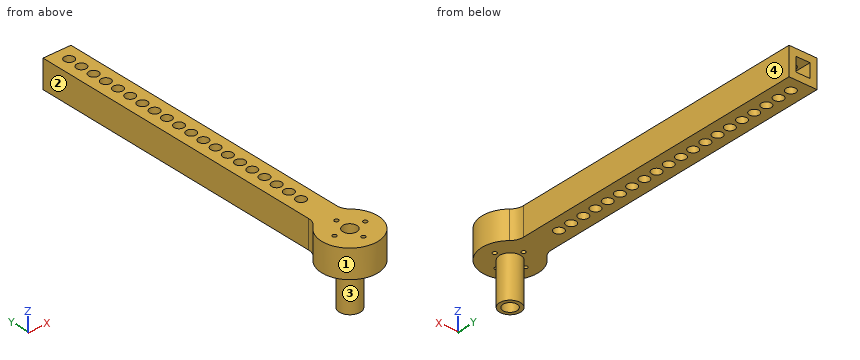
```python
from build123d import *

# Parameters (mm, degrees)
SKETCH1_W           = 12.7
SKETCH1_H           = 12.7
SKETCH1_W_2         = 6.35
SKETCH1_H_2         = 6.35
BOSS_EXTRUDE1_DEPTH = 152.4
SKETCH2_R           = 2.226999991
CUT_EXTRUDE1_DEPTH  = 13.7
SKETCH3_R           = 12.7
BOSS_EXTRUDE2_DEPTH = 12.7
SKETCH4_R           = 4.7625
BOSS_EXTRUDE3_DEPTH = 31.75
SKETCH6_R           = 3.175
SKETCH6_R_2         = 0.927000051
CUT_EXTRUDE3_DEPTH  = 32.75
FILLET2_R           = 6.35


with BuildPart() as part:
    # Sketch1 → Boss-Extrude1 (new body)
    with BuildSketch(Plane(origin=(0, 0, 0), x_dir=(1, 0, 0), z_dir=(0, 1, 0))):
        Rectangle(SKETCH1_W, SKETCH1_H)
        Rectangle(SKETCH1_W_2, SKETCH1_H_2, mode=Mode.SUBTRACT)
    extrude(amount=BOSS_EXTRUDE1_DEPTH)

    # Sketch2 → Cut-Extrude1 (cut, through all)
    with BuildSketch(Plane.XY.offset(6.35)):
        with Locations((0, 25.4)):
            Circle(SKETCH2_R)
        with Locations((0, 31.75)):
            Circle(SKETCH2_R)
        with Locations((0, 38.1)):
            Circle(SKETCH2_R)
        with Locations((0, 44.45)):
            Circle(SKETCH2_R)
        with Locations((0, 50.8)):
            Circle(SKETCH2_R)
        with Locations((0, 57.15)):
            Circle(SKETCH2_R)
        with Locations((0, 63.5)):
            Circle(SKETCH2_R)
        with Locations((0, 69.85)):
            Circle(SKETCH2_R)
        with Locations((0, 76.2)):
            Circle(SKETCH2_R)
        with Locations((0, 82.55)):
            Circle(SKETCH2_R)
        with Locations((0, 88.9)):
            Circle(SKETCH2_R)
        with Locations((0, 95.25)):
            Circle(SKETCH2_R)
        with Locations((0, 101.6)):
            Circle(SKETCH2_R)
        with Locations((0, 107.95)):
            Circle(SKETCH2_R)
        with Locations((0, 114.3)):
            Circle(SKETCH2_R)
        with Locations((0, 120.65)):
            Circle(SKETCH2_R)
        with Locations((0, 127)):
            Circle(SKETCH2_R)
        with Locations((0, 133.35)):
            Circle(SKETCH2_R)
        with Locations((0, 139.7)):
            Circle(SKETCH2_R)
        with Locations((0, 146.05)):
            Circle(SKETCH2_R)
    extrude(amount=-CUT_EXTRUDE1_DEPTH, mode=Mode.SUBTRACT)

    # Sketch3 → Boss-Extrude2 (add)
    with BuildSketch(Plane.XY.offset(6.35)):
        Circle(SKETCH3_R)
    extrude(amount=-BOSS_EXTRUDE2_DEPTH)

    # Sketch4 → Boss-Extrude3 (add)
    with BuildSketch(Plane.XY.offset(6.35)):
        Circle(SKETCH4_R)
    extrude(amount=-BOSS_EXTRUDE3_DEPTH)

    # Sketch6 → Cut-Extrude3 (cut, through all)
    with BuildSketch(Plane.XY.offset(6.35)):
        Circle(SKETCH6_R)
        with Locations((6.99999997, 0)):
            Circle(SKETCH6_R_2)
        with Locations((0, -6.99999997)):
            Circle(SKETCH6_R_2)
        with Locations((-6.99999997, 0)):
            Circle(SKETCH6_R_2)
        with Locations((0, 6.99999997)):
            Circle(SKETCH6_R_2)
    extrude(amount=-CUT_EXTRUDE3_DEPTH, mode=Mode.SUBTRACT)

    # Fillet2
    fillet2_edges = [part.edges().sort_by_distance(p)[0] for p in [
        (6.35, 10.998522628, 0),
        (-6.35, 10.998522628, 0),
    ]]
    fillet(fillet2_edges, radius=FILLET2_R)


solid = part.part
```
CAD build for the part. Positions are in the model's coordinates, mm. Face numbers are marked on the shaded views. A direction names the side the tool comes from. Give positions to 0.01 mm unless a question says otherwise; leave off trailing zeros. Write each loop counter-clockwise with the first axis right and the second up, starting at its lowest first coordinate (ties: lowest second). Pieces come first, ordered by that corner, then holes. Notation, with made-up numbers: M 46.5,41.5 L 67.5,41.5 A25 cw 67.5,62.5 Z; hole C 42.5,-18 d4. An arc over 180 degrees is marked long. Return JSON: item names as keys, results as strings. Group by question number.
(1) 3-axis set-ups, long thin cutter, end or side, ignore diameter. For the marked faces 1, 2, 3 and 4: which of +Z, -Z, +X, -X, +Y, -Y reach the whole face in a straight line?
(2) Band-saw the part on A-A (y = 20). Give the cut face in (x, z) (3 decimals), and give its area (3 significant figures).
(3) Band-saw the part on B-B (y = 50.8). Give the cut face in (x, z) (3 decimals), and give its area (3 significant figures).
(4) Flat gauge pins, fed straight in: pin 1 Ø1.5 at (x, z) = (3.5, -8.5) entering from +Y; pin 2 Ø2.5 at (x, y) = (0, 76.2) entering from -Z; pin 3 Ø10 at (y, z) = (91, 0.5) entering from +X; pin 4 Ø3 at (x, z) = (-1.5, -13) entering from +Y. Where does each tip first touch, or does it go through?
(5) Drill centre lines: L1, parallel to Y at x = -0.25, z = -0.5; L2, parallel to X at y = 112.5, z = -1.5 (3 decimals). Where is each one in solid material? Low to high. Write a range as [from, to].
Entries:
{
 "1": {"face 1": "+Z, -Z", "face 2": "+Z, -Z, -X, +Y", "face 3": "-Z", "face 4": "+Z, -Z, +X, +Y"},
 "2": {"outline": "M -6.35,-6.35 L 6.35,-6.35 L 6.35,6.35 L -6.35,6.35 Z; hole M -3.175,-3.175 L 3.175,-3.175 L 3.175,3.175 L -3.175,3.175 Z", "area": "121 mm^2"},
 "3": {"outline": "M -6.35,-6.35 L -2.227,-6.35 L -2.227,-3.175 L -3.175,-3.175 L -3.175,3.175 L -2.227,3.175 L -2.227,6.35 L -6.35,6.35 Z; M 2.227,-6.35 L 6.35,-6.35 L 6.35,6.35 L 2.227,6.35 L 2.227,3.175 L 3.175,3.175 L 3.175,-3.175 L 2.227,-3.175 Z", "area": "92.7 mm^2"},
 "4": {"pin 1": "stops at y = 3.89", "pin 2": "passes through", "pin 3": "stops at x = 6.35", "pin 4": "stops at y = 4.76"},
 "5": {"L1": "y = [-12.7, -7.89], [-6.11, -3.17], [3.17, 6.11], [7.89, 12.7]", "L2": "x = [-6.35, -3.175], [3.175, 6.35]"}
}
